Autodesk Inventor part; units mm, degrees
ref_plane "YZ Plane" through (0, 0, 0) normal (1, 0, 0) x (0, 1, 0)
ref_plane "XZ Plane" through (0, 0, 0) normal (0, 1, 0) x (-1, 0, 0)
ref_plane "XY Plane" through (0, 0, 0) normal (0, 0, 1) x (1, 0, 0)
sketch "Esboço1" plane through (0, 0, 0) normal (0, 1, 0) x (-1, 0, 0)
  line L0 (-18.5, 20) -> (18.5, 20)
  line L1 (20, 18.5) -> (20, -18.5)
  line L2 (18.5, -20) -> (-18.5, -20)
  line L3 (-20, -18.5) -> (-20, 18.5)
  line L4 (-20, 20) -> (20, -20) construction
  line L5 (20, 20) -> (-20, -20) construction
  line L6 (-18.5, -18.5) -> (18.5, -18.5)
  line L7 (18.5, -18.5) -> (18.5, 18.5)
  line L8 (18.5, 18.5) -> (-18.5, 18.5)
  line L9 (-18.5, 18.5) -> (-18.5, -18.5)
  line L10 (-18.5, -18.5) -> (18.5, 18.5) construction
  line L11 (18.5, -18.5) -> (-18.5, 18.5) construction
  arc A0 (20, 18.5) -> (18.5, 20) centre (18.5, 18.5) ccw
  arc A1 (-18.5, 20) -> (-20, 18.5) centre (-18.5, 18.5) ccw
  arc A2 (-20, -18.5) -> (-18.5, -20) centre (-18.5, -18.5) ccw
  arc A3 (18.5, -20) -> (20, -18.5) centre (18.5, -18.5) ccw
  point P0 (0, 0)
  dimension "d0" = 40
  dimension "d1" = 40
  dimension "d2" = 1.5
  dimension "d3" = 1.5
extrude "Extrusão1" add sketch "Esboço1" along normal mid plane 700
equation "\"d3\" = d2"
properties part number "MSI-101" material "Aço inoxidável AISI 304"
Work out the finished part from the listing and answer in its coordinate system (mm). A direction names the side the tool comes from. Give positions to 0.01 mm unless a question says otherwise; leave off trailing zeros. Order: outer loops, then holes, each group sorted by start corner. A loop starts at its lowest first (then second) coordinate and runs counter-clockwise, first axis right, second up. Notation, with made-up numbers: (76.5, 58) -> (126.5, 58) arc R27 ccw to (126.5, 84) -> close; hole circle Ø9 at (22, -10). An arc over 180 degrees is marked (long way). Answer as a JSON object with one key per item and string values. Group by question number.
1. Section B-B on y = -20.5 is taken. Determine the outline of the cut face in (x, z).
2. Section C-C on z = -9 is taken. Determine the outline of the cut face in (x, y).
3. Section A-A on x = 0 is taken. Determine the outline of the cut face in (y, z).
4. Consider line 1 along X through (y, z) = (-149, 14.5). Determine where the line is inside the solid, lowest interval first. Write a range as [from, to].
5. A flat-ended cylindrical pin translates along its axis: pin 1 Ø3 at (x, z) = (-16, 14.5) entering from -Y. Find the tip coordinate at first contact, or state that the pin passes through.
6. The mould has two halves that part along X. Classify faces 1 (the flat face through (-20, -5, 0)), 2 (the flat face through (20, -5, 0)), 3 (the flat face through (2, 350, -19)), 4 (the flat face through (0, -5, -18.5)): released by +X, released by -X, zero draft, split by the parting line, or undercut.
7. A tool of negligible diameter and unlimited length cuts with its end or side. For faces 5 (the flat face through (0, -5, -20)), 6 (the flat face through (0, -5, 18.5)), from which of +Z, -Z, +X, -X, +Y, -Y can it reach the whole face along a straight path? Write none if from no direction.
Result sheet:
{
 "1": {"outline": "(-20, -18.5) arc R1.5 ccw to (-18.5, -20) -> (18.5, -20) arc R1.5 ccw to (20, -18.5) -> (20, 18.5) arc R1.5 ccw to (18.5, 20) -> (-18.5, 20) arc R1.5 ccw to (-20, 18.5) -> close; hole (-18.5, -18.5) -> (18.5, -18.5) -> (18.5, 18.5) -> (-18.5, 18.5) -> close"},
 "2": {"outline": "(-20, -350) -> (-18.5, -350) -> (-18.5, 350) -> (-20, 350) -> close; (18.5, -350) -> (20, -350) -> (20, 350) -> (18.5, 350) -> close"},
 "3": {"outline": "(-350, -20) -> (350, -20) -> (350, -18.5) -> (-350, -18.5) -> close; (-350, 18.5) -> (350, 18.5) -> (350, 20) -> (-350, 20) -> close"},
 "4": {"line 1": "x = [-20, -18.5], [18.5, 20]"},
 "5": {"pin 1": "passes through"},
 "6": {"face 1": "released by -X", "face 2": "released by +X", "face 3": "zero draft", "face 4": "undercut"},
 "7": {"face 5": "-Z, +X, -X, +Y, -Y", "face 6": "+Y, -Y"}
}
